Verification items for this drawing (mm, ordinates from the low corner). A direction names the side the tool comes from. Coordinates: 2 decimals unless noted, no trailing zeros. Loops run counter-clockwise (first coordinate to the right, second up) from the corner with the lowest first, then second, coordinate; pieces in that order, holes last. Notation, with made-up numbers: M 26,41.5 L 34,41.5 A34 ccw 34,75.5 Z; hole C 73,12 d5. An arc over 180 degrees is marked long. Return JSON: item names as keys, results as strings.
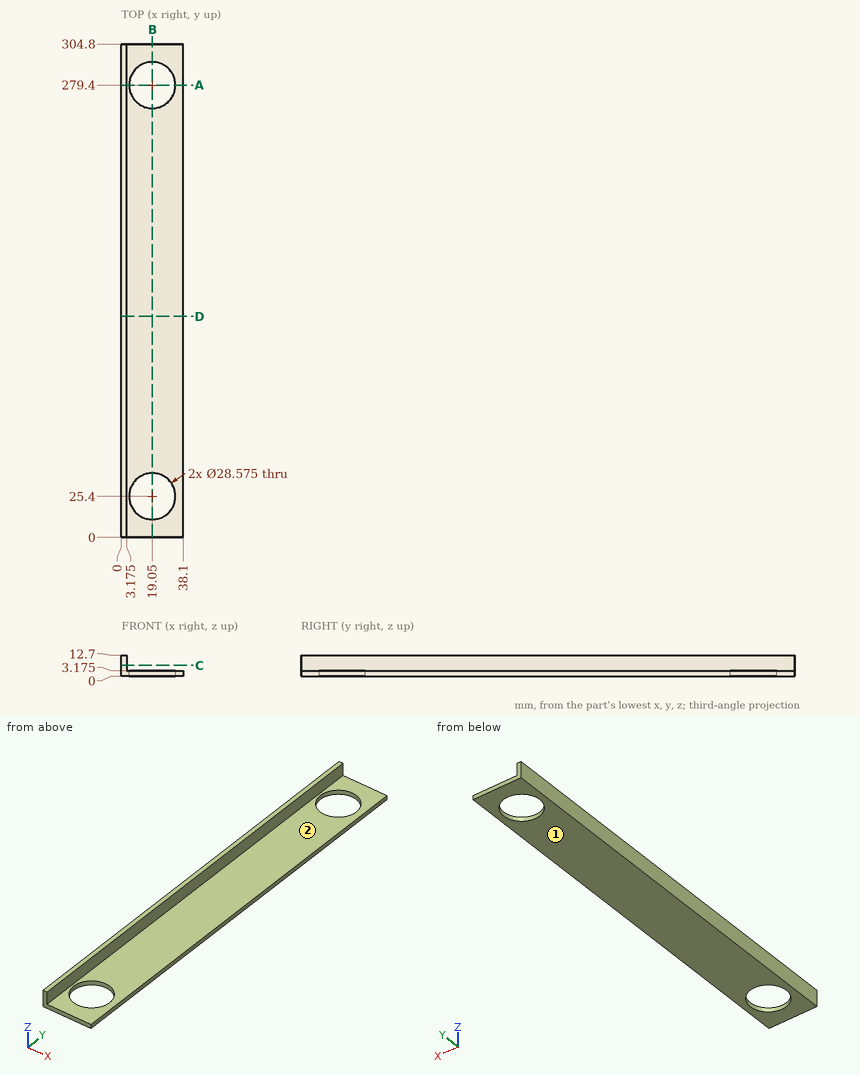
1) Go/stop test with flat-tipped pins: pin 1 Ø1 at (x, z) = (10.5, 3.5) entering from +Y; pin 2 Ø3 at (x, y) = (6.5, 200.5) entering from +Z (3 decimals). Record where each tip stops, or that it passes through.
Answers:
{"pin 1": "y = 304.8", "pin 2": "z = 3.175"}
2) Section check D-D on y = 136.5. Record the cut outline in (x, z) (3 decimals).
Answers:
{"outline": "M 0,0 L 38.1,0 L 38.1,3.175 L 3.175,3.175 L 3.175,12.7 L 0,12.7 Z"}
3) Scan lines: line 1 along Y through (x, z) = (19.05, 0.95); line 2 along Z through (x, y) = (30, 67) (3 decimals). Record each from-to range of solid material in increasing order. Write a range as [from, to].
Answers:
{"line 1": "[0, 11.11], [39.69, 265.11], [293.69, 304.8]", "line 2": "[0, 3.175]"}
4) Set-up check for the marked faces 1 and 2: record each of +Z, -Z, +X, -X, +Y, -Y from which the full face is reachable in a straight line by a thin tool's end or side.
Answers:
{"face 1": "-Z, +X, -X, +Y, -Y", "face 2": "+Z, +X, +Y, -Y"}
5) Section check C-C on z = 6.5. Record the cut outline in (x, y) (3 decimals).
Answers:
{"outline": "M 0,0 L 3.175,0 L 3.175,304.8 L 0,304.8 Z"}
6) Section check A-A on y = 279.4. Record the cut outline in (x, z) (1 decimal), then the cut area to 3 significant figures.
Answers:
{"outline": "M 0,0 L 4.8,0 L 4.8,3.2 L 3.2,3.2 L 3.2,12.7 L 0,12.7 Z; M 33.3,0 L 38.1,0 L 38.1,3.2 L 33.3,3.2 Z", "area": "60.5 mm²"}
7) Section check B-B on x = 19.05. Record the cut outline in (y, z) (1 decimal), then the cut area to 3 significant figures.
Answers:
{"outline": "M 0,0 L 11.1,0 L 11.1,3.2 L 0,3.2 Z; M 39.7,0 L 265.1,0 L 265.1,3.2 L 39.7,3.2 Z; M 293.7,0 L 304.8,0 L 304.8,3.2 L 293.7,3.2 Z", "area": "786 mm²"}
